Autodesk Inventor part; units mm, degrees
ref_plane "YZ Plane" through (0, 0, 0) normal (1, 0, 0) x (0, 1, 0)
ref_plane "XZ Plane" through (0, 0, 0) normal (0, 1, 0) x (-1, 0, 0)
ref_plane "XY Plane" through (0, 0, 0) normal (0, 0, 1) x (1, 0, 0)
sketch "Sketch1" plane through (0, 0, 0) normal (0, 0, 1) x (1, 0, 0)
  line L0 (-64, 50) -> (64, 50)
  line L1 (64, 50) -> (64, 0)
  line L2 (64, 0) -> (-64, 0)
  line L3 (-64, 0) -> (-64, 50)
  line L4 (-25, 0) -> (25, 0)
  line L5 (25, 0) -> (25, -2)
  line L6 (25, -2) -> (-25, -2)
  line L7 (-25, -2) -> (-25, 0)
  point P0 (0, 0)
  point P1 (0, 0)
  dimension "d0" = 128
  dimension "d1" = 50
  dimension "d2" = 50
  dimension "d3" = 2
extrude "Extrusion1" add sketch "Sketch1" along normal mid plane 2
sketch "Sketch2" plane through (0, 0, 1) normal (0, 0, 1) x (1, 0, 0)
  line L0 (53.9533, 19.1647) -> (54.2948, 15.001)
  line L1 (54.2948, 15.001) -> (-55.3369, 6.0072)
  line L2 (-55.3369, 6.0072) -> (-55.6784, 10.1709)
  line L3 (-55.6784, 10.1709) -> (53.9533, 19.1647)
  line L4 (62.1376, 13.5765) -> (61.7855, 17.8679)
  line L5 (-63.1946, 7.615) -> (-62.8426, 3.3235)
  point P0 (0, 0)
sketch "Sketch3" plane through (0, 0, 1) normal (0, 0, 1) x (1, 0, 0)
  line L0 (-62.8426, 9.5832) -> (61.6275, 19.7943)
  line L1 (-55.6784, 10.1709) -> (53.9533, 19.1647)
  line L2 (-63.1946, 7.615) -> (-62.8426, 3.3235) construction
  line L3 (62.1376, 13.5765) -> (61.7855, 17.8679) construction
  line L4 (-62.8426, 9.5832) -> (-62.8426, 0)
  line L5 (-64, 0) -> (-25, 0)
  line L6 (61.6275, 19.7943) -> (61.6275, 0)
  line L7 (61.6275, 19.7943) -> (62.7021, 6.6951) construction
  line L8 (-62.8426, 0) -> (-72.8426, 0)
  line L9 (-72.8426, 0) -> (-72.8426, 60)
  line L10 (-72.8426, 60) -> (71.6275, 60)
  line L11 (71.6275, 60) -> (71.6275, 0)
  line L12 (71.6275, 0) -> (61.6275, 0)
  point P0 (0, 0)
  dimension "d6" = 10
  dimension "d7" = 10
  dimension "d8" = 60
extrude "Extrusion2" cut sketch "Sketch3" against normal through all
sketch "Sketch4" plane through (0, 0, 1) normal (0, 0, 1) x (1, 0, 0)
  line L0 (56, 0) -> (56, 19.4013)
  line L1 (54, 0) -> (56, 0)
  line L2 (54, 19.4013) -> (54, 0)
  line L3 (54, 19.4013) -> (56, 19.4013)
  line L4 (-54, 0) -> (-54, 10.4075)
  line L5 (-56, 0) -> (-54, 0)
  line L6 (-56, 10.4075) -> (-56, 0)
  line L7 (-56, 10.4075) -> (-54, 10.4075)
  point P0 (0, 0)
sketch "Sketch5" plane through (0, 0, 1) normal (0, 0, 1) x (1, 0, 0)
  line L0 (-56, 10.4075) -> (-56, 0) construction
  line L1 (-54, 0) -> (-54, 10.4075) construction
  line L2 (54, 19.4013) -> (54, 0) construction
  line L3 (56, 0) -> (56, 19.4013) construction
  line L4 (-54, 4) -> (-56, 4)
  line L5 (-56, 4) -> (-56, 24)
  line L6 (-56, 24) -> (-54, 24)
  line L7 (-54, 24) -> (-54, 4)
  line L8 (56, 24) -> (54, 24)
  line L9 (54, 24) -> (54, 4)
  line L10 (54, 4) -> (56, 4)
  line L11 (56, 4) -> (56, 24)
  line L12 (25, 0) -> (61.6275, 0)
  line L13 (-62.8426, 0) -> (-25, 0)
  point P0 (0, 0)
  dimension "d11" = 4
  dimension "d12" = 20
  dimension "d13" = 4
  dimension "d14" = 20
extrude "Extrusion3" cut sketch "Sketch5" against normal through all
properties part number "angle_plate_long_tall"
Could you check a few things on this model? Use its own coordinates, in mm. A direction names the side the tool comes from. Round coordinates to 2 decimals unless told otherwise and drop trailing zeros. Write each loop counter-clockwise with the first axis right and the second up, starting at its lowest first coordinate (ties: lowest second). Pieces come first, ordered by that corner, then holes. Notation, with made-up numbers: M 64,7 L 105,7 A21 cw 105,11 Z; hole C -36,44.5 d9. An arc over 180 degrees is marked long. Answer in a Markdown table with one row per item. Add a question column.
Q1. Imagine slicing it at D-D (x = -31.5). Please give me the cut outline in (y, z).
Q2. Imagine slicing it at A-A (y = 13). Please give me the cut outline in (x, z), then the cut area to 3 significant figures.
Q3. Imagine slicing it at B-B (y = 8). Please give me the cut outline in (x, z).
Q4. Will these pins go through, and if not, where does the flat tip stop? pin 1 Ø1 at (x, z) = (42.5, -0.5) entering from -Y; pin 2 Ø0.6 at (y, z) = (-1, -0.5) entering from +X.
Q5. Imagine slicing it at C-C (z = 0.5). Please give me the cut outline in (x, y).
Q6. If I drill on line 1 (X direction, y = 8.5, z = 0.8); line 2 (Y direction, x = 55, z = 0.95); line 3 (Y direction, x = -33.5, z = 0.8), over which ranges is the centre line in solid material (lowest first)? Write a range as from..to.
Q7. On a 3-axis mill with a long thin cutter (end or side, diameter ignored), from which of +Z, -Z, +X, -X, +Y, -Y can I reach the whole of each face in a straight line? I mean faces 1 (the flat face through (-25, -1, 0)), 2 (the flat face through (54, 12, 0)), 3 (the flat face through (25, -1, 0)). Say none if no direction works.
Q8. If we mould it in two halves opening along X, with no side actions, what happens to faces 4 (the flat face through (61.628, 10, 0)), 5 (the flat face through (-44, 0, 0)), 6 (the flat face through (-54, 7, 0)), 7 (the flat face through (-62.843, 5, 0))? For each: +X half, -X half, draft (parallel to the pull), parting line (faces both ways), or undercut.
Values:
| question | item | result |
|---|---|---|
| 1 | outline | M 0,-1 L 12.15,-1 L 12.15,1 L 0,1 Z |
| 2 | outline | M -21.19,-1 L 54,-1 L 54,1 L -21.19,1 Z; M 56,-1 L 61.63,-1 L 61.63,1 L 56,1 Z |
| 2 | area | 162 mm^2 |
| 3 | outline | M -62.84,-1 L -56,-1 L -56,1 L -62.84,1 Z; M -54,-1 L 54,-1 L 54,1 L -54,1 Z; M 56,-1 L 61.63,-1 L 61.63,1 L 56,1 Z |
| 4 | pin 1 | y = 0 |
| 4 | pin 2 | x = 25 |
| 5 | outline | M -62.84,0 L -25,0 L -25,-2 L 25,-2 L 25,0 L 61.63,0 L 61.63,19.79 L 56,19.33 L 56,4 L 54,4 L 54,19.17 L -54,10.31 L -54,4 L -56,4 L -56,10.14 L -62.84,9.58 Z |
| 6 | line 1 | -62.84..-56, -54..54, 56..61.63 |
| 6 | line 2 | 0..4 |
| 6 | line 3 | 0..11.99 |
| 7 | face 1 | +Z, -Z, -X, -Y |
| 7 | face 2 | +Z, -Z, +Y |
| 7 | face 3 | +Z, -Z, +X, -Y |
| 8 | face 4 | +X half |
| 8 | face 5 | draft |
| 8 | face 6 | undercut |
| 8 | face 7 | -X half |
